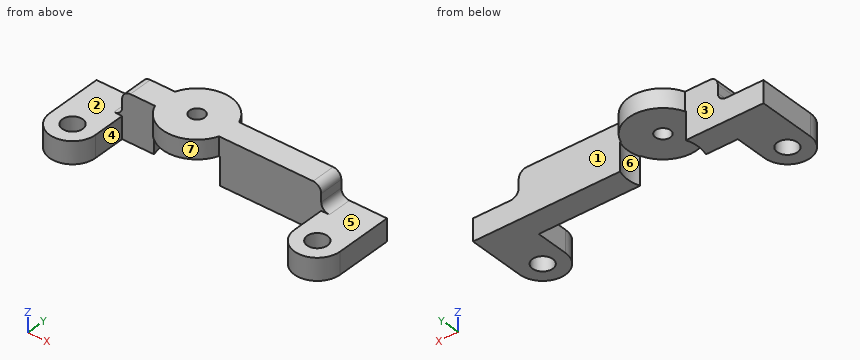
from build123d import *

# Parameters (mm, degrees)
SKETCH_1_R          = 1.25
SKETCH_1_R_2        = 0.925
EXTRUDE_1_DEPTH     = 7.7
SKETCH_2_R          = 4.3
CUT_EXTRUDE_1_DEPTH = 3.4
CUT_EXTRUDE_2_DEPTH = 5
CUT_EXTRUDE_3_DEPTH = 2
FILLET_2_R          = 1


with BuildPart() as part:
    # 草图1 → 凸台-拉伸1 (new body)
    with BuildSketch(Plane.XY):
        with BuildLine():
            Line((-8.173009049, 0.432285115), (-12.2, 0.432285115))
            Line((-12.2, 0.432285115), (-17.8, 0.432285115))
            Line((-17.8, 0.432285115), (-17.8, -6.567714885))
            ThreePointArc((-17.8, -6.567714885), (-15, -9.367714885), (-12.2, -6.567714885))
            Line((-12.2, -6.567714885), (-12.2, -3.067714885))
            Line((-12.2, -3.067714885), (-12.2, -2.567714885))
            Line((-12.2, -2.567714885), (-8.173009049, -2.567714885))
            ThreePointArc((-8.173009049, -2.567714885), (-4.25, -5.267714885), (-0.326990951, -2.567714885))
            Line((-0.326990951, -2.567714885), (12.2, -2.567714885))
            Line((12.2, -2.567714885), (12.2, -6.567714885))
            ThreePointArc((12.2, -6.567714885), (15, -9.367714885), (17.8, -6.567714885))
            Line((17.8, -6.567714885), (17.8, 0.432285115))
            Line((17.8, 0.432285115), (12.2, 0.432285115))
            Line((12.2, 0.432285115), (-0.326990951, 0.432285115))
            ThreePointArc((-0.326990951, 0.432285115), (-4.25, 3.132285115), (-8.173009049, 0.432285115))
        make_face()
        with Locations((-15, -6.567714885)):
            Circle(SKETCH_1_R, mode=Mode.SUBTRACT)
        with Locations((15, -6.567714885)):
            Circle(SKETCH_1_R, mode=Mode.SUBTRACT)
        with Locations((-4.25, -1.067714885)):
            Circle(SKETCH_1_R_2, mode=Mode.SUBTRACT)
        with BuildLine():
            Line((-8.173009049, 0.432285115), (-12.2, 0.432285115))
            Line((-12.2, 0.432285115), (-17.8, 0.432285115))
            Line((-17.8, 0.432285115), (-17.8, -6.567714885))
            ThreePointArc((-17.8, -6.567714885), (-15, -9.367714885), (-12.2, -6.567714885))
            Line((-12.2, -6.567714885), (-12.2, -3.067714885))
            Line((-12.2, -3.067714885), (-12.2, -2.567714885))
            Line((-12.2, -2.567714885), (-8.173009049, -2.567714885))
            ThreePointArc((-8.173009049, -2.567714885), (-4.25, -5.267714885), (-0.326990951, -2.567714885))
            Line((-0.326990951, -2.567714885), (12.2, -2.567714885))
            Line((12.2, -2.567714885), (12.2, -6.567714885))
            ThreePointArc((12.2, -6.567714885), (15, -9.367714885), (17.8, -6.567714885))
            Line((17.8, -6.567714885), (17.8, 0.432285115))
            Line((17.8, 0.432285115), (12.2, 0.432285115))
            Line((12.2, 0.432285115), (-0.326990951, 0.432285115))
            ThreePointArc((-0.326990951, 0.432285115), (-4.25, 3.132285115), (-8.173009049, 0.432285115))
        make_face()
        with Locations((-15, -6.567714885)):
            Circle(SKETCH_1_R, mode=Mode.SUBTRACT)
        with Locations((15, -6.567714885)):
            Circle(SKETCH_1_R, mode=Mode.SUBTRACT)
        with Locations((-4.25, -1.067714885)):
            Circle(SKETCH_1_R_2, mode=Mode.SUBTRACT)
    extrude(amount=EXTRUDE_1_DEPTH)

    # 草图2 → 切除-拉伸1 (cut)
    with BuildSketch(Plane(origin=(0, 0, 0), x_dir=(-1, 0, 0), z_dir=(0, 0, -1))):
        with Locations((4.25, -1.067714885)):
            Circle(SKETCH_2_R)
    extrude(amount=-CUT_EXTRUDE_1_DEPTH, mode=Mode.SUBTRACT)

    # 草图3 → 切除-拉伸2 (cut)
    with BuildSketch(Plane.XY.offset(7.7)):
        with BuildLine():
            Line((-17.8, 0.432285115), (-12.2, 0.432285115))
            Line((-12.2, 0.432285115), (-12.2, -6.567714885))
            ThreePointArc((-12.2, -6.567714885), (-15, -9.367714885), (-17.8, -6.567714885))
            Line((-17.8, -6.567714885), (-17.8, 0.432285115))
        make_face()
        with BuildLine():
            Line((12.2, 0.432285115), (17.8, 0.432285115))
            Line((17.8, 0.432285115), (17.8, -6.567714885))
            ThreePointArc((17.8, -6.567714885), (15, -9.367714885), (12.2, -6.567714885))
            Line((12.2, -6.567714885), (12.2, 0.432285115))
        make_face()
    extrude(amount=-CUT_EXTRUDE_2_DEPTH, mode=Mode.SUBTRACT)

    # 草图5 → 切除-拉伸3 (cut)
    with BuildSketch(Plane.XY.offset(7.7)):
        with BuildLine():
            Line((12.2, -2.567714885), (-0.326990951, -2.567714885))
            ThreePointArc((-0.326990951, -2.567714885), (-4.25, -5.267714885), (-8.173009049, -2.567714885))
            Line((-8.173009049, -2.567714885), (-12.2, -2.567714885))
            Line((-12.2, -2.567714885), (-12.2, 0.432285115))
            Line((-12.2, 0.432285115), (-8.173009049, 0.432285115))
            ThreePointArc((-8.173009049, 0.432285115), (-4.25, 3.132285115), (-0.326990951, 0.432285115))
            Line((-0.326990951, 0.432285115), (12.2, 0.432285115))
            Line((12.2, 0.432285115), (12.2, -2.567714885))
        make_face()
    extrude(amount=-CUT_EXTRUDE_3_DEPTH, mode=Mode.SUBTRACT)

    # 圆角2
    fillet_2_edges = [part.edges().sort_by_distance(p)[0] for p in [
        (12.2, -1.067714885, 5.7),
        (-12.2, -1.067714885, 5.7),
        (-12.2, -1.067714885, 2.7),
        (12.2, -1.067714885, 2.7),
    ]]
    fillet(fillet_2_edges, radius=FILLET_2_R)


solid = part.part
Verification items for the finished model (mm, model axes). Face numbers are marked on the shaded views. A direction names the side the tool comes from. Give positions to 0.01 mm unless a question says otherwise; leave off trailing zeros. Loops run counter-clockwise (first coordinate to the right, second up) from the corner with the lowest first, then second, coordinate; pieces in that order, holes last.
1. Material ranges on probe 1 along Y at (x, z) = (-15, 1.5); probe 2 along X at (y, z) = (-3, 1.5); probe 3 along Z at (x, y) = (15, -4.75), recorded low to high.
Derived:
probe 1: y = -9.37 to -7.82, -5.32 to 0.43
probe 2: x = -17.8 to -12.2, 12.2 to 17.8
probe 3: z = 0 to 2.7
2. Go/stop test with flat-tipped pins: P1, Ø2.5, axis at x = -11.5, z = 4, coming from the -Y side; P2, Ø1.1, axis at y = -1.5, z = 4, coming from the -X side; P3, Ø6, axis at x = -15.5, y = -5, coming from the +Z side; P4, Ø2, axis at x = 8, y = 1.5, coming from the +Z side. Record where each tip stops, or that it passes through.
Derived:
P1: stops at y = -2.57
P2: stops at x = -12.23
P3: stops at z = 2.7
P4: passes through
3. Cross-section at B-B on y = -4. Record the cut outline in (x, z), and give its area (3 significant figures).
Derived:
outline: (-17.8, 0) - (-12.2, 0) - (-12.2, 2.7) - (-17.8, 2.7) - close; (-7.26, 3.4) - (-1.24, 3.4) - (-1.24, 5.7) - (-7.26, 5.7) - close; (12.2, 0) - (17.8, 0) - (17.8, 2.7) - (12.2, 2.7) - close
area: 44.1 mm2
4. Release check for a two-part mould opening along Y. For the marked faces 5, 6 and 7 record: +Y half, -Y half, draft (parallel to the pull), parting line (faces both ways), or undercut.
Derived:
face 5: draft
face 6: undercut
face 7: -Y half
5. Tool access check on the marked faces 1, 2, 3 and 4. Record the directions out of +Z, -Z, +X, -X, +Y, -Y that give a thin tool (end or side, any length) a straight path to the whole face; none if there is none.
Derived:
face 1: +Z, -Z, +X, +Y
face 2: +Z, -X, -Y
face 3: +Z, -Z, -X, +Y
face 4: +Z, -Z, -Y
6. Cross-section at C-C on x = -4.25. Record the cut outline in (y, z).
Derived:
outline: (-5.27, 3.4) - (-1.99, 3.4) - (-1.99, 5.7) - (-5.27, 5.7) - close; (-0.14, 3.4) - (3.13, 3.4) - (3.13, 5.7) - (-0.14, 5.7) - close
7. Cross-section at A-A on x = -15. Record the cut outline in (y, z).
Derived:
outline: (-9.37, 0) - (-7.82, 0) - (-7.82, 2.7) - (-9.37, 2.7) - close; (-5.32, 0) - (0.43, 0) - (0.43, 2.7) - (-5.32, 2.7) - close
